from build123d import *

# Parameters (mm, degrees)
SKETCH1_W                = 29.21
SKETCH1_H                = 29.21
BOSS_EXTRUDE1_DEPTH      = 41.91
SKETCH2_W                = 14.732
SKETCH2_H                = 14.732
CUT_EXTRUDE1_DEPTH       = 8.255
SKETCH3_W                = 24.13
SKETCH3_H                = 19.05
CUT_EXTRUDE2_DEPTH       = 33.655
SKETCH6_W                = 4.699
SKETCH6_H                = 4.445
CUT_EXTRUDE3_DEPTH       = 4.445
BOSS_EXTRUDE2_DEPTH      = 27.94
FILLET1_R                = 10
CHAMFER2_SIZE            = 5.08
CUT_EXTRUDE4_DEPTH       = 27.94
CUT_EXTRUDE5_DEPTH       = 16.51
BOSS_EXTRUDE3_DEPTH      = 10.16
M6_CLEARANCE_HOLE1_D     = 6.8032
M6_CLEARANCE_HOLE1_DEPTH = 32.5000112
M6_CLEARANCE_HOLE1_TIP   = 2.043887482
SKETCH18_W               = 12.7
SKETCH18_H               = 16.067158518
CUT_EXTRUDE9_DEPTH       = 12.7
BOSS_EXTRUDE4_DEPTH      = 3.81
SKETCH19_W               = 5.08
SKETCH19_H               = 5.08
CUT_EXTRUDE10_DEPTH      = 8.89


with BuildPart() as part:
    # Sketch1 → Boss-Extrude1 (new body)
    with BuildSketch(Plane(origin=(0, 0, 0), x_dir=(1, 0, 0), z_dir=(0, 1, 0))):
        Rectangle(SKETCH1_W, SKETCH1_H)
    extrude(amount=BOSS_EXTRUDE1_DEPTH)

    # Sketch2 → Cut-Extrude1 (cut)
    with BuildSketch(Plane.XZ):
        Rectangle(SKETCH2_W, SKETCH2_H)
    extrude(amount=-CUT_EXTRUDE1_DEPTH, mode=Mode.SUBTRACT)

    # Sketch3 → Cut-Extrude2 (cut)
    with BuildSketch(Plane.XZ.offset(-8.255)):
        Rectangle(SKETCH3_W, SKETCH3_H)
    extrude(amount=-CUT_EXTRUDE2_DEPTH, mode=Mode.SUBTRACT)

    # Sketch6 → Cut-Extrude3 (cut)
    with BuildSketch(Plane(origin=(0, 8.255, 0), x_dir=(1, 0, 0), z_dir=(0, 1, 0))):
        with Locations((-9.7155, 0)):
            Rectangle(SKETCH6_W, SKETCH6_H)
    cut_extrude3 = extrude(amount=-CUT_EXTRUDE3_DEPTH, mode=Mode.SUBTRACT)

    # Mirror1: Cut-Extrude3 across plane
    add(cut_extrude3.mirror(Plane(origin=(0, 0, 0), x_dir=(0, 0, 1), z_dir=(1, 0, 0))), mode=Mode.SUBTRACT)

    # Sketch7 → Boss-Extrude2 (add)
    with BuildSketch(Plane(origin=(0, 41.91, 0), x_dir=(1, 0, 0), z_dir=(0, 1, 0))):
        with BuildLine():
            Line((-14.605, -2.997916359), (-35.433403696, -2.997916359))
            ThreePointArc((-35.433403696, -2.997916359), (0, -35.56), (35.433403696, -2.997916359))
            Line((35.433403696, -2.997916359), (14.605, -2.997916359))
            Line((14.605, -2.997916359), (14.605, -14.605))
            Line((14.605, -14.605), (-14.605, -14.605))
            Line((-14.605, -14.605), (-14.605, -2.997916359))
        make_face()
        Polygon((-12.065, -2.997916359), (-14.605, -2.997916359), (-14.605, -14.605), (14.605, -14.605), (14.605, -2.997916359), (12.065, -2.997916359), (12.065, -9.525), (-12.065, -9.525), align=None)
    extrude(amount=BOSS_EXTRUDE2_DEPTH)

    # Fillet1
    fillet1_edges = [part.edges().sort_by_distance(p)[0] for p in [
        (-13.335, 41.91, 2.997916359),
        (13.335, 41.91, 2.997916359),
    ]]
    fillet(fillet1_edges, radius=FILLET1_R)

    # Chamfer2
    chamfer2_edges = [part.edges().sort_by_distance(p)[0] for p in [
        (0, 0, 14.605),
        (-14.605, 0, 0),
        (0, 0, -14.605),
        (14.605, 0, 0),
    ]]
    chamfer(chamfer2_edges, length=CHAMFER2_SIZE)

    # Sketch8 → Cut-Extrude4 (cut)
    with BuildSketch(Plane(origin=(0, 69.85, 0), x_dir=(1, 0, 0), z_dir=(0, 1, 0))):
        with BuildLine():
            Line((-14.605, -2.997916359), (-35.433403696, -2.997916359))
            ThreePointArc((-35.433403696, -2.997916359), (-32.258645828, -14.963066843), (-25.174526181, -25.114872716))
            Line((-25.174526181, -25.114872716), (-14.605, -6.807916359))
            Line((-14.605, -6.807916359), (-14.605, -2.997916359))
        make_face()
    cut_extrude4 = extrude(amount=-CUT_EXTRUDE4_DEPTH, mode=Mode.SUBTRACT)

    # Mirror2: Cut-Extrude4 across plane
    add(cut_extrude4.mirror(Plane(origin=(0, 0, 0), x_dir=(0, 0, 1), z_dir=(1, 0, 0))), mode=Mode.SUBTRACT)

    # Sketch9 → Cut-Extrude5 (cut)
    with BuildSketch(Plane.XZ.offset(-41.91)):
        with BuildLine():
            Line((-14.605, 6.807916359), (-14.605, 14.605))
            Line((-14.605, 14.605), (14.605, 14.605))
            Line((14.605, 14.605), (14.605, 6.807916359))
            Line((14.605, 6.807916359), (25.174526181, 25.114872716))
            ThreePointArc((25.174526181, 25.114872716), (0, 35.56), (-25.174526181, 25.114872716))
            Line((-25.174526181, 25.114872716), (-14.605, 6.807916359))
        make_face()
    extrude(amount=-CUT_EXTRUDE5_DEPTH, mode=Mode.SUBTRACT)

    # Sketch11 → Boss-Extrude3 (add)
    with BuildSketch(Plane(origin=(0, 58.42, 0), x_dir=(-1, 0, 0), z_dir=(0, -1, 0))):
        with BuildLine():
            Line((14.605, -6.807916359), (14.605, -14.605))
            Line((14.605, -14.605), (-14.605, -14.605))
            Line((-14.605, -14.605), (-14.605, -6.807916359))
            Line((-14.605, -6.807916359), (-21.525014254, -18.793732635))
            ThreePointArc((-21.525014254, -18.793732635), (0, -28.575), (21.525014254, -18.793732635))
            Line((21.525014254, -18.793732635), (14.605, -6.807916359))
        make_face()
    extrude(amount=BOSS_EXTRUDE3_DEPTH)

    # M6 Clearance Hole1
    with Locations(Plane(origin=(0, 69.85, 0), x_dir=(1, 0, 0), z_dir=(0, 1, 0))):
        with Locations((0, -15.399579259)):
            Hole(M6_CLEARANCE_HOLE1_D / 2, depth=M6_CLEARANCE_HOLE1_DEPTH)
            with Locations((0, 0, -(M6_CLEARANCE_HOLE1_DEPTH + M6_CLEARANCE_HOLE1_TIP / 2))):  # 118° drill point
                Cone(0, M6_CLEARANCE_HOLE1_D / 2, M6_CLEARANCE_HOLE1_TIP, mode=Mode.SUBTRACT)

    # Sketch18 → Cut-Extrude9 (cut)
    with BuildSketch(Plane.XZ.offset(-48.26)):
        with Locations((0, 15.399579259)):
            Rectangle(SKETCH18_W, SKETCH18_H)
    extrude(amount=CUT_EXTRUDE9_DEPTH, mode=Mode.SUBTRACT)

    # Sketch14 → Boss-Extrude4 (add)
    with BuildSketch(Plane.ZY.offset(14.605)):
        Polygon((14.605, 48.26), (20.955, 48.26), (14.605, 31.75), align=None)
    boss_extrude4 = extrude(amount=-BOSS_EXTRUDE4_DEPTH)

    # Mirror3: Boss-Extrude4 across plane
    add(boss_extrude4.mirror(Plane(origin=(0, 0, 0), x_dir=(0, 0, 1), z_dir=(1, 0, 0))))

    # Sketch19 → Cut-Extrude10 (cut)
    with BuildSketch(Plane(origin=(0, 41.91, 0), x_dir=(1, 0, 0), z_dir=(0, 1, 0))):
        with Locations((0, 12.065)):
            Rectangle(SKETCH19_W, SKETCH19_H)
    extrude(amount=-CUT_EXTRUDE10_DEPTH, mode=Mode.SUBTRACT)


solid = part.part
Part model, mm, in its own coordinate system. A direction names the side the tool comes from. Give positions to 0.01 mm unless a question says otherwise; leave off trailing zeros. Loops run counter-clockwise (first coordinate to the right, second up) from the corner with the lowest first, then second, coordinate; pieces in that order, holes last. Notation, with made-up numbers: M 63.25,78.25 L 115.25,78.25 A14 cw 115.25,105.25 Z; hole C 50.25,27 d5. An arc over 180 degrees is marked long. Put each result on its own line as item: value. Start each with the question number.
1) Saw through at B-B (y = 28.5). List the corners of the cut face in (x, z) (3 decimals).
2) Saw through at A-A (x = 0). List the corners of the cut face in (y, z) (3 decimals), then the cut area to 3 significant figures.
3) Saw through at D-D (x = -16). List the corners of the cut face in (y, z).
4) Probe probe 1 along X at (y, z) = (18, -3) (3 decimals); probe 2 along Z at (x, y) = (0, 64) (3 decimals); probe 3 along Z at (x, y) = (0, 53) (3 decimals). List the from-to ranges inside material, lowest first.
5) Pull direction Z, two halves, no side cores. Call faces 1 (the flat face through (13, 61, 2.998)), 2 (the flat face through (0, 58.42, 29)), 3 (the flat face through (10, 3.81, 0)): +Z half, -Z half, draft (parallel to the pull), parting line (faces both ways), or undercut.
6) Saw through at C-C (z = -1). List the corners of the cut face in (x, y) (3 decimals).
7) 3-axis set-ups, long thin cutter, end or side, ignore diameter. For faces 4 (the flat face through (0, 8.255, 8)), 5 (the flat face through (10.795, 44, 16)), 6 (the flat face through (-6.35, 42, 12)), 7 (the flat face through (0, 33.02, -12)): which of +Z, -Z, +X, -X, +Y, -Y reach the whole face in a straight line?
8) Flat gauge pins, fed straight in: pin 1 (8 mm diameter, centred on y = 36.5, z = 15, fed in from -X) (3 decimals); pin 2 (2 mm diameter, centred on x = -5.5, z = 5.5, fed in from -Y); pin 3 (3.5 mm diameter, centred on x = -10.5, y = 5.5, fed in from +Z) (3 decimals); pin 4 (4 mm diameter, centred on y = 36, z = -11, fed in from +X) (3 decimals). Where does each tip first touch, or does it go through?
Numbers:
1. outline: M -14.605,-14.605 L 14.605,-14.605 L 14.605,14.605 L -14.605,14.605 Z; hole M -12.065,-9.525 L 12.065,-9.525 L 12.065,9.525 L -12.065,9.525 Z
2. outline: M 0,-9.525 L 5.08,-14.605 L 33.02,-14.605 L 33.02,-9.525 L 8.255,-9.525 L 8.255,-7.366 L 0,-7.366 Z; M 0,7.366 L 8.255,7.366 L 8.255,9.525 L 35.56,9.525 L 35.56,14.605 L 5.08,14.605 L 0,9.525 Z; M 48.26,9.525 L 69.85,9.525 L 69.85,11.998 L 48.26,11.998 Z; M 48.26,18.801 L 69.85,18.801 L 69.85,35.56 L 58.42,35.56 L 58.42,28.575 L 48.26,28.575 Z
2. area: 702 mm^2
3. outline: M 48.26,9.22 L 69.85,9.22 L 69.85,31.76 L 58.42,31.76 L 58.42,23.68 L 48.26,23.68 Z
4. probe 1: -14.605 to -12.065, 12.065 to 14.605
4. probe 2: 9.525 to 11.998, 18.801 to 35.56
4. probe 3: 9.525 to 11.998, 18.801 to 28.575
5. face 1: -Z half
5. face 2: draft
5. face 3: undercut
6. outline: M -14.605,5.08 L -9.525,0 L -7.366,0 L -7.366,3.81 L -12.065,3.81 L -12.065,43.912 L -14.605,43.912 Z; M 7.366,0 L 9.525,0 L 14.605,5.08 L 14.605,43.912 L 12.065,43.912 L 12.065,3.81 L 7.366,3.81 Z
7. face 4: +Y
7. face 5: +Z, -Y
7. face 6: +Z
7. face 7: -Z, +Y
8. pin 1: x = -14.605
8. pin 2: through
8. pin 3: z = 14.605
8. pin 4: x = 14.605
